Check sheet for the modelled part. Datum: model origin and axes. Units: mm. A direction names the side the tool comes from. Give positions to 0.01 mm unless a question says otherwise; leave off trailing zeros. Loops run counter-clockwise (first coordinate to the right, second up) from the corner with the lowest first, then second, coordinate; pieces in that order, holes last. Notation, with made-up numbers: M -32.75,35 L -26.75,35 A22 ccw -26.75,46 Z; hole C -38.5,-26.5 d6. An arc over 180 degrees is marked long. Use one line per item in the form item = value.
from build123d import *

# Parameters (mm, degrees)
EXTRUDE_THIN2_DEPTH            = 22
SKETCH3_W                      = 44
SKETCH3_H                      = 44
CUT_EXTRUDE1_DEPTH             = 0.7625
SKETCH4_R                      = 10.1
CUT_EXTRUDE2_DEPTH             = 5
F_8_32_TAPPED_HOLE1_AT_2_COUNT = 2
F_8_32_TAPPED_HOLE1_AT_2_PITCH = 26.846787517
F_8_32_TAPPED_HOLE1_AT_3_COUNT = 2
F_8_32_TAPPED_HOLE1_AT_3_PITCH = 26.846787517
CHAMFER2_SIZE                  = 0.5
FILLET1_R                      = 1


with BuildPart() as part:
    # Sketch2 → Extrude-Thin2 (new body, symmetric)
    with BuildSketch(Plane(origin=(0, 0, 0), x_dir=(1, 0, 0), z_dir=(0, 1, 0))):
        Polygon((0, -50.8), (0, 0), (-50.8, 0), (-50.8, -4.7625), (-4.7625, -4.7625), (-4.7625, -50.8), align=None)
    extrude(amount=EXTRUDE_THIN2_DEPTH, both=True)

    # Sketch3 → Cut-Extrude1 (cut)
    with BuildSketch(Plane.ZY.offset(4.7625)):
        with Locations((28.8, 0)):
            Rectangle(SKETCH3_W, SKETCH3_H)
    extrude(amount=-CUT_EXTRUDE1_DEPTH, mode=Mode.SUBTRACT)

    # Sketch4 → Cut-Extrude2 (cut, through all)
    with BuildSketch(Plane.ZY.offset(4)):
        with Locations((28.8, 0)):
            Circle(SKETCH4_R)
    extrude(amount=-CUT_EXTRUDE2_DEPTH, mode=Mode.SUBTRACT)

    # Sketch6 → #8-32 Tapped Hole1 (revolve, cut)
    with BuildSketch(Plane(origin=(-4, 15.5, 28.8), x_dir=(0, 0, 1), z_dir=(0, 1, 0))):
        Polygon((0, 0), (0, 4), (2.7178, 4), (1.7272, 3.0094), (1.7272, 0.9906), (2.7178, 0), align=None)
    f_8_32_tapped_hole1 = revolve(axis=Axis((-10.35, 15.5, 28.8), (1, 0, 0)), mode=Mode.SUBTRACT)

    # #8-32 Tapped Hole1 at 2: #8-32 Tapped Hole1 ×2
    with Locations(*[Vector(0, -0.866025404, 0.5) * (i * F_8_32_TAPPED_HOLE1_AT_2_PITCH) for i in range(1, F_8_32_TAPPED_HOLE1_AT_2_COUNT)]):
        add(f_8_32_tapped_hole1, mode=Mode.SUBTRACT)

    # #8-32 Tapped Hole1 at 3: #8-32 Tapped Hole1 ×2
    with Locations(*[Vector(0, -0.866025404, -0.5) * (i * F_8_32_TAPPED_HOLE1_AT_3_PITCH) for i in range(1, F_8_32_TAPPED_HOLE1_AT_3_COUNT)]):
        add(f_8_32_tapped_hole1, mode=Mode.SUBTRACT)

    # Chamfer2
    chamfer2_edges = [part.edges().sort_by_distance(p)[0] for p in [
        (0, 0, 18.7),
        (-4, 0, 18.7),
    ]]
    chamfer(chamfer2_edges, length=CHAMFER2_SIZE)

    # Fillet1
    fillet1_edges = [part.edges().sort_by_distance(p)[0] for p in [
        (0, 22, 25.4),
        (-25.4, 22, 0),
        (-50.8, 22, 2.38125),
        (-27.78125, 22, 4.7625),
        (-4, -22, 28.8),
        (-4, 0, 50.8),
        (-4, 22, 28.8),
        (-27.78125, -22, 4.7625),
        (-50.8, -22, 2.38125),
        (-25.4, -22, 0),
        (0, -22, 25.4),
        (-2, -22, 50.8),
        (-2, 22, 50.8),
        (-50.8, 0, 4.7625),
        (-50.8, 0, 0),
        (0, 0, 0),
        (0, 0, 50.8),
    ]]
    fillet(fillet1_edges, radius=FILLET1_R)


solid = part.part
1) Set-up check for faces 4 (the face through (-2.021, 3.034, 38.434)), 5 (the face through (-4, 5, 18)): record each of +Z, -Z, +X, -X, +Y, -Y from which the full face is reachable in a straight line by a thin tool's end or side.
Evaluation:
face_4 = +X, -X
face_5 = +Z, -X, +Y, -Y
2) Section check A-A (z = 28.8). Record the cut outline in (x, y), then the cut area to 3 significant figures.
Evaluation:
outline = M -4,-21 A1 ccw -3,-22 L -1,-22 A1 ccw 0,-21 L 0,-10.6 L -0.5,-10.1 L -3.5,-10.1 L -4,-10.6 Z; M -4,10.6 L -3.5,10.1 L -0.5,10.1 L 0,10.6 L 0,12.78 L -0.99,13.77 L -3.01,13.77 L -4,12.78 Z; M -4,18.22 L -3.01,17.23 L -0.99,17.23 L 0,18.22 L 0,21 A1 ccw -1,22 L -3,22 A1 ccw -4,21 Z
area = 78.1 mm^2
3) Section check B-B (y = 0). Record the cut outline in (x, z), then the cut area to 3 significant figures.
Evaluation:
outline = M -50.8,1 A1 ccw -49.8,0 L -1,0 A1 ccw 0,1 L 0,18.2 L -0.5,18.7 L -3.5,18.7 L -4,18.2 L -4,6.8 L -4.76,6.8 L -4.76,4.76 L -49.8,4.76 A1 ccw -50.8,3.76 Z; M -4,39.4 L -3.5,38.9 L -0.5,38.9 L 0,39.4 L 0,49.8 A1 ccw -1,50.8 L -3,50.8 A1 ccw -4,49.8 Z
area = 345 mm^2
4) Depth check by flat-ended pin: pin 1 Ø4 at (y, z) = (15.5, 28.8) entering from +X; pin 2 Ø5 at (x, z) = (-34, 7) entering from -Y; pin 3 Ø4 at (x, y) = (-21, -14) entering from +Z; pin 4 Ø3 at (y, z) = (-7.75, 15.38) entering from +X. Enter the tip coordinate at first touch or a pass-through.
Evaluation:
pin_1 = -0.72
pin_2 = -21.68
pin_3 = 4.76
pin_4 = through
5) Section check D-D (z = 9). Record the cut outline in (x, y).
Evaluation:
outline = M -4,-21 A1 ccw -3,-22 L -1,-22 A1 ccw 0,-21 L 0,21 A1 ccw -1,22 L -3,22 A1 ccw -4,21 Z
6) Release check for a two-part mould opening along Z. For faces 1 (the face through (0, 0, 15)), 2 (the face through (-2.014, 13.787, 28.575)), 3 (the face through (-28, 0, 4.762)) record: pulls with the +Z half, pulls with the -Z half, needs draft (parallel to the pull), parting line crosses it, or undercut.
Evaluation:
face_1 = needs draft
face_2 = undercut
face_3 = pulls with the +Z half
7) Scan lines: line 1 (Y direction, x = -1.9, z = 28.8); line 2 (Z direction, x = -1.45, y = 15.5); line 3 (X direction, y = -12, z = 28.5). Record each from-to range of solid material in increasing order.
Evaluation:
line_1 = -22 to -10.1, 10.1 to 13.77, 17.23 to 22
line_2 = 0 to 27.07, 30.53 to 50.8
line_3 = -4 to 0
8) Section check C-C (x = -28). Record the cut outline in (y, z).
Evaluation:
outline = M -22,1 A1 ccw -21,0 L 21,0 A1 ccw 22,1 L 22,3.76 A1 ccw 21,4.76 L -21,4.76 A1 ccw -22,3.76 Z
